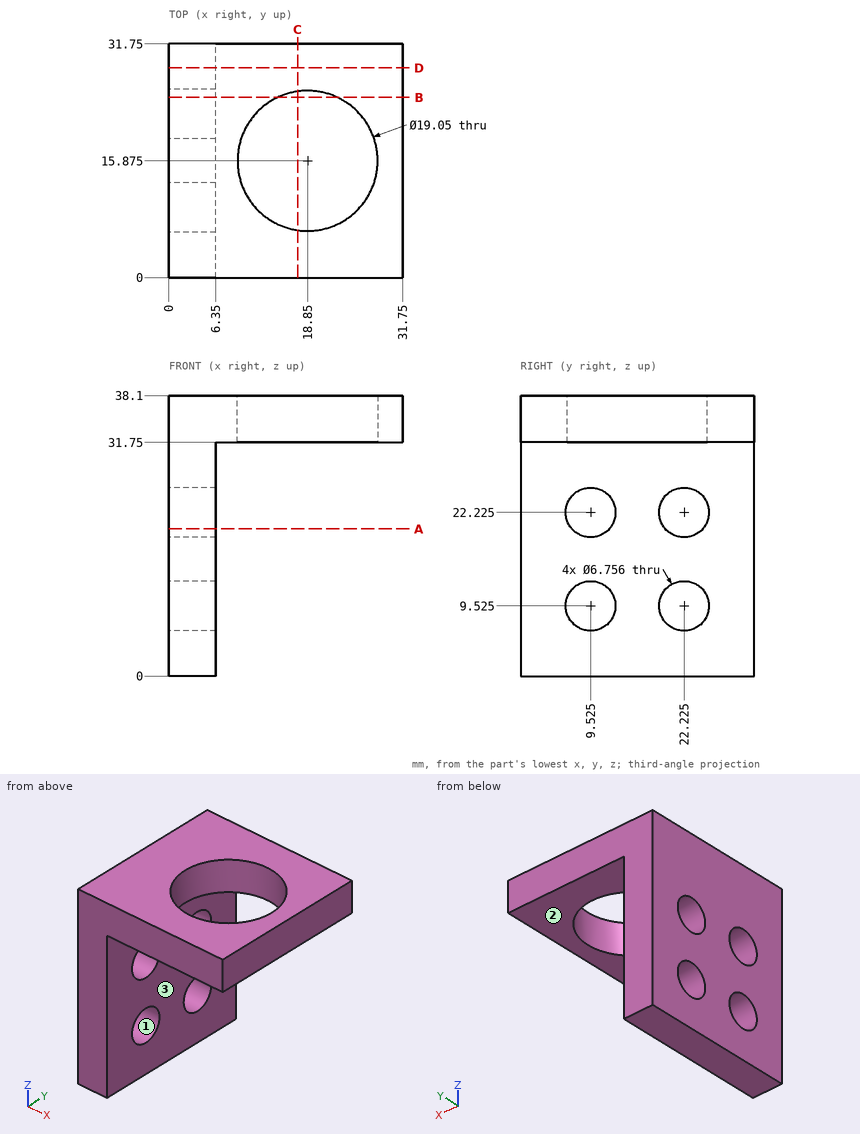
Design review of the part shown in the three views and the two pictorial views. Dimensions are in mm from the part's minimum x, y and z. Round coordinates to 2 decimals unless told otherwise and drop trailing zeros. Write each loop counter-clockwise with the first axis right and the second up, starting at its lowest first coordinate (ties: lowest second). Pieces come first, ordered by that corner, then holes. Notation, with made-up numbers: M 16,32.5 L 40,32.5 A16 cw 40,48.5 Z; hole C -25,17 d9. An arc over 180 degrees is marked long. Use a Markdown table: item, result. Add a question column.
Q1. Insertion check: pin 1 (12.5 mm diameter, centred on x = 17.5, y = 16.5, fed in from -Z); pin 2 (8 mm diameter, centred on y = 22.225, z = 22.225, fed in from +X). Each pin has a flat end and moves straight along its axis. Give the tip position at first contact, or say it passes through.
Q2. To check wall thickness, follow line 1 (Z direction, x = 3.5, y = 25); line 2 (Z direction, x = 28.5, y = 4); line 3 (X direction, y = 13, z = 29). State the ranges of each line that lie inside material, in increasing order.
Q3. We need section A-A, the plane z = 20. State the section outline as (x, y) points, plus the area to 3 significant figures.
Q4. The part is to be moulded in two halves that separate along Z. For the marked faces 1, 2 and 3, say which applies: pulls with the +Z half, pulls with the -Z half, needs draft (parallel to the pull), parting line crosses it, or undercut.
Q5. We need section D-D, the plane y = 28.5. State the section outline as (x, z) points, plus the area to 3 significant figures.
Q6. We need section B-B, the plane y = 24.5. State the section outline as (x, z) points.
Q7. We need section C-C, the plane x = 17.5. State the section outline as (y, z) points.
Findings below:
| question | item | result |
|---|---|---|
| 1 | pin 1 | passes through |
| 1 | pin 2 | stops at x = 6.35 |
| 2 | line 1 | z = 0 to 7.6, 11.45 to 20.3, 24.15 to 38.1 |
| 2 | line 2 | z = 31.75 to 38.1 |
| 2 | line 3 | x = 0 to 6.35 |
| 3 | outline | M 0,0 L 6.35,0 L 6.35,6.98 L 0,6.98 Z; M 0,12.07 L 6.35,12.07 L 6.35,19.68 L 0,19.68 Z; M 0,24.77 L 6.35,24.77 L 6.35,31.75 L 0,31.75 Z |
| 3 | area | 137 mm² |
| 4 | face 1 | undercut |
| 4 | face 2 | pulls with the -Z half |
| 4 | face 3 | needs draft |
| 5 | outline | M 0,0 L 6.35,0 L 6.35,31.75 L 31.75,31.75 L 31.75,38.1 L 0,38.1 Z |
| 5 | area | 403 mm² |
| 6 | outline | M 0,0 L 6.35,0 L 6.35,7.03 L 0,7.03 Z; M 0,12.02 L 6.35,12.02 L 6.35,19.73 L 0,19.73 Z; M 0,24.72 L 6.35,24.72 L 6.35,31.75 L 14.81,31.75 L 14.81,38.1 L 0,38.1 Z; M 22.89,31.75 L 31.75,31.75 L 31.75,38.1 L 22.89,38.1 Z |
| 7 | outline | M 0,31.75 L 6.45,31.75 L 6.45,38.1 L 0,38.1 Z; M 25.3,31.75 L 31.75,31.75 L 31.75,38.1 L 25.3,38.1 Z |
